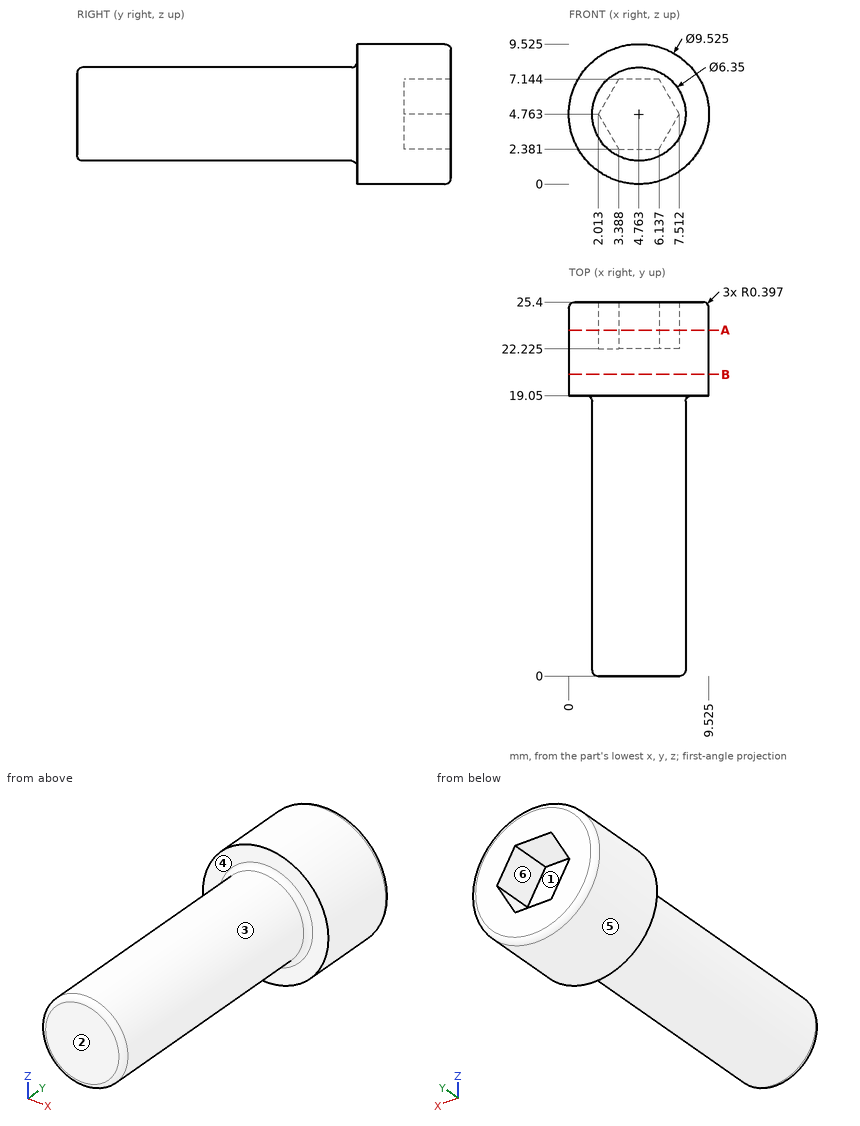
Input: dimensioned drawing with shaded views. Units: mm. Origin: part minimum x, y, z. A direction names the side the tool comes from. Give positions to 0.01 mm unless a question says otherwise; leave off trailing zeros. Write each loop counter-clockwise with the first axis right and the second up, starting at its lowest first coordinate (ties: lowest second). Pieces come first, ordered by that corner, then holes.
1. Section query A-A (y = 23.5). Return the cut outline in (x, z) (1 decimal).
2. Pull-direction query (Z, two-part tool) for the marked faces 1, 2 and 3; classes: +Z half, -Z half, draft (parallel to the pull), parting line (faces both ways), or undercut.
3. Access query for the marked faces 4, 5 and 6. Directions: +Z, -Z, +X, -X, +Y, -Y. A direction counts if a zero-diameter tool reaches every point of the face in a straight line with its end or side. Return the directions, or none.
4. First-contact query: pin 1 (2.5 mm diameter, centred on x = 5, z = 4, fed in from +Y) (1 decimal); pin 2 (2 mm diameter, centred on x = 6.5, y = 17.5, fed in from -Z) (1 decimal); pin 3 (2 mm diameter, centred on y = 13.5, z = 4.5, fed in from -X). Flat tips, straight axial feed; report the tip coordinate or a pass-through.
5. Section query B-B (y = 20.5). Return the cut outline in (x, z) (1 decimal).
6. Material intervals for line 1 along Y through (x, z) = (3.75, 4.75) (1 decimal); line 2 along Y through (x, z) = (1.75, 7); line 3 along X through (y, z) = (23.75, 4.5) (1 decimal), sorted ascending.
Output values:
1. outline: circle Ø9.5 at (4.8, 4.8); hole (2, 4.8) - (3.4, 2.4) - (6.1, 2.4) - (7.5, 4.8) - (6.1, 7.1) - (3.4, 7.1) - close
2. face 1: undercut
2. face 2: draft
2. face 3: parting line
3. face 4: -Y
3. face 5: +Y, -Y
3. face 6: +Y
4. pin 1: stops at y = 22.2
4. pin 2: stops at z = 1.7
4. pin 3: stops at x = 1.59
5. outline: circle Ø9.5 at (4.8, 4.8)
6. line 1: y = 0 to 22.2
6. line 2: y = 19.05 to 25.4
6. line 3: x = 0 to 2.2, 7.4 to 9.5
